Here's the drawing with two shaded views (mm, measured from the low corner). I have some questions. A direction names the side the tool comes from. Round coordinates to 2 decimals unless told otherwise and drop trailing zeros. Write each loop counter-clockwise with the first axis right and the second up, starting at its lowest first coordinate (ties: lowest second). Pieces come first, ordered by that corner, then holes. Notation, with made-up numbers: M 87.5,59 L 95.5,59 A23 ccw 95.5,97 Z; hole C -8.5,18 d3. An arc over 180 degrees is marked long. Write item = value, one per line. Start each with the question number.
(1) If we mould it in two halves opening along Z, with no side actions, what happens to the marked faces 1, 2 and 3? For each: released by +Z, released by -Z, zero draft, split by the parting line, or undercut.
(2) Will these pins go through, and if not, where does the flat tip stop? pin 1 Ø0.9 at (x, y) = (15, 2) entering from +Z; pin 2 Ø1 at (y, z) = (0.5, 30) entering from -X.
(3) I want a section at B-B (x = 7.5). List the corners of the cut face in (y, z) for me, and give its area (3 significant figures).
(4) I want a section at C-C (y = 0.9). List the corners of the cut face in (x, z) for me, and give its area (3 significant figures).
(5) I want a section at D-D (x = 19.75). List the corners of the cut face in (y, z) for me.
(6) I want a section at A-A (z = 8.5). List the corners of the cut face in (x, y) for me, and give its area (3 significant figures).
(7) I need wall thicknesses on line 1 along X through (y, z) = (2, 16); line 2 along Z through (x, y) = (16.25, 1.65); line 3 along X through (y, z) = (4, 14). Which ranges of each line are inside material? Lowest first, please.
(8) On a 3-axis mill with a long thin cutter (end or side, diameter ignored), from which of +Z, -Z, +X, -X, +Y, -Y can I reach the whole of each face in a straight line? I mean the marked faces 4 and 5. Say none if no direction works.
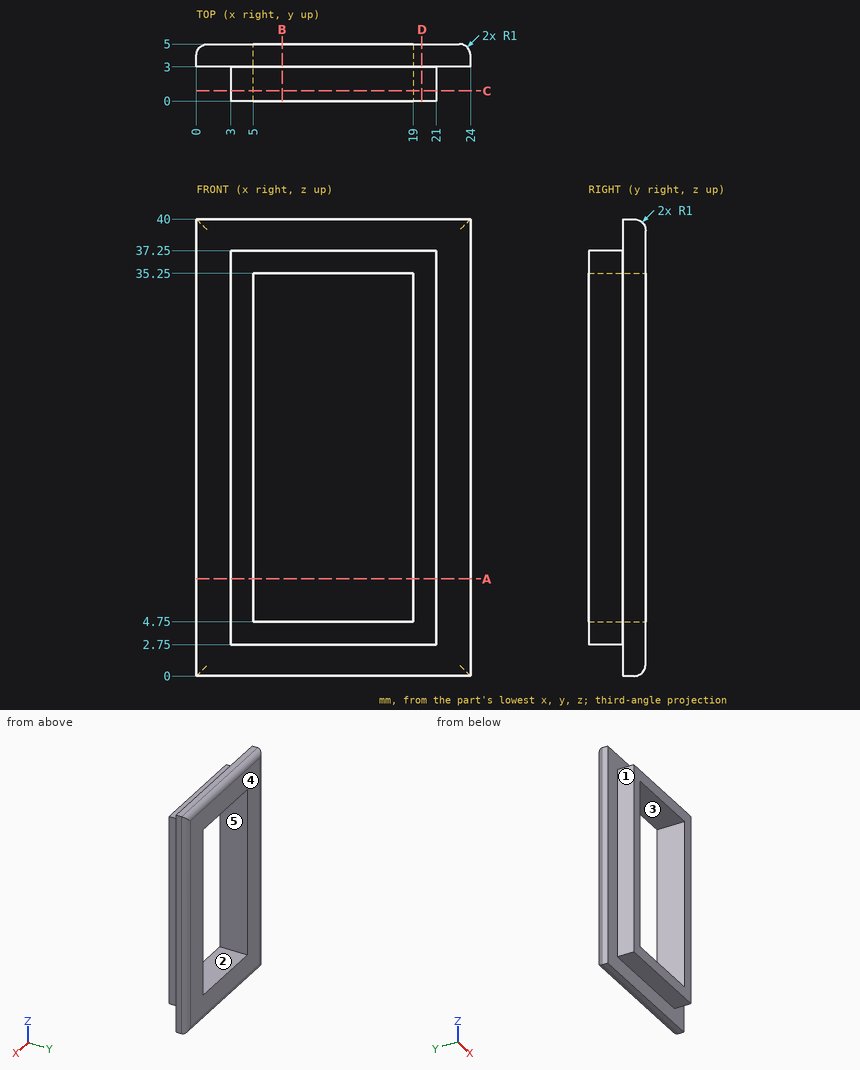
Returned:
q1.face_1 = zero draft
q1.face_2 = undercut
q1.face_3 = undercut
q2.pin_1 = 37.25
q2.pin_2 = 3
q3.outline = M 0,2.75 L 3,2.75 L 3,0 L 4,0 A1 ccw 5,1 L 5,4.75 L 0,4.75 Z; M 0,35.25 L 5,35.25 L 5,39 A1 ccw 4,40 L 3,40 L 3,37.25 L 0,37.25 Z
q3.area = 30.6 mm²
q4.outline = M 3,2.75 L 21,2.75 L 21,37.25 L 3,37.25 Z; hole M 5,4.75 L 19,4.75 L 19,35.25 L 5,35.25 Z
q4.area = 194 mm²
q5.outline = M 0,2.75 L 3,2.75 L 3,0 L 4,0 A1 ccw 5,1 L 5,39 A1 ccw 4,40 L 3,40 L 3,37.25 L 0,37.25 Z
q6.outline = M 0,3 L 3,3 L 3,0 L 5,0 L 5,5 L 1,5 A1 ccw 0,4 Z; M 19,0 L 21,0 L 21,3 L 24,3 L 24,4 A1 ccw 23,5 L 19,5 Z
q6.area = 31.6 mm²
q7.line_1 = 3 to 5, 19 to 21
q7.line_2 = 2.75 to 4.75, 35.25 to 37.25
q7.line_3 = 0 to 5, 19 to 24
q8.face_4 = +Z, -Z, +X, -X, +Y
q8.face_5 = +Y, -Y
